Work out the finished part from the listing and answer in its coordinate system (mm). A direction names the side the tool comes from. Give positions to 0.01 mm unless a question says otherwise; leave off trailing zeros. Loops run counter-clockwise (first coordinate to the right, second up) from the corner with the lowest first, then second, coordinate; pieces in that order, holes last. Notation, with made-up numbers: M 26.5,33.5 L 61.5,33.5 A24 ccw 61.5,51.5 Z; hole C 34.5,2.25 d4. An arc over 180 degrees is marked long. Use a Markdown table: item, result.
Autodesk Inventor part; units mm, degrees
ref_plane "YZ Plane" through (0, 0, 0) normal (1, 0, 0) x (0, 1, 0)
ref_plane "XZ Plane" through (0, 0, 0) normal (0, 1, 0) x (-1, 0, 0)
ref_plane "XY Plane" through (0, 0, 0) normal (0, 0, 1) x (1, 0, 0)
sketch "Sketch1" plane through (0, 0, 0) normal (0, 0, 1) x (1, 0, 0)
  circle A0 centre (0, 0) radius 10.16
  line L0 (3.7395, -6.477) -> (-3.7395, -6.477)
  line L1 (-3.7395, -6.477) -> (-7.479, 0)
  line L2 (-7.479, 0) -> (-3.7395, 6.477)
  line L3 (-3.7395, 6.477) -> (3.7395, 6.477)
  line L4 (3.7395, 6.477) -> (7.479, 0)
  line L5 (7.479, 0) -> (3.7395, -6.477)
  dimension "d0" = 20.32
  dimension "d1" = 12.954
extrude "Extrusion1" add sketch "Sketch1" along normal blind 5.7112
properties part number "3DPRINT,KICKER,MOTOR,SPACER" material "ABS Plastic"
(1) The mould has two halves that part along X. Classify faces 3 (the flat face through (0, -7, 0)), 4 (the flat face through (-5.583, -3.284, 2.816)), 5 (the cylindrical face through (-1.323, -10.074, 2.816)), 6 (the flat face through (5.635, -3.193, 2.816)): released by +X, released by -X, zero draft, split by the parting line, or undercut.
Entries:
| item | result |
|---|---|
| face 3 | zero draft |
| face 4 | undercut |
| face 5 | split by the parting line |
| face 6 | undercut |
(2) Consider probe 1 along X at (y, z) = (1.75, 4.9); probe 2 along X at (y, z) = (-0.25, 0.5); probe 3 along Y at (x, z) = (6, 0.75). Determine where each line is inside the solid, lowest interval first. Write a range as [from, to].
Entries:
| item | result |
|---|---|
| probe 1 | x = [-10.01, -6.47], [6.47, 10.01] |
| probe 2 | x = [-10.16, -7.33], [7.33, 10.16] |
| probe 3 | y = [-8.2, -2.56], [2.56, 8.2] |
(3) Which of the six approach directions +Z, -Z, +X, -X, +Y, -Y give full straight-line access (tool end or side, diameter ignored) to faces 1 (the flat face through (-5.635, 3.193, 2.816)), 2 (the flat face through (0, -7, 5.711))?
Entries:
| item | result |
|---|---|
| face 1 | +Z, -Z |
| face 2 | +Z, +X, -X, +Y, -Y |
(4) Given P1, Ø2, axis at x = 3, z = 2, coming from the -Y side; P2, Ø4, axis at x = 3, y = -2.5, coming from the -Z side; P3, Ø1.5, axis at x = -4.5, z = 4, coming from the -Y side, each flat-ended and moving along its own axis, determine where each tip first touches the part or whether it passes through.
Entries:
| item | result |
|---|---|
| P1 | stops at y = -9.96 |
| P2 | passes through |
| P3 | stops at y = -9.44 |
(5) A cutting plane is placed at D-D (x = 9.25). Write down the section's boundary in (y, z), and give its area (3 significant figures).
Entries:
| item | result |
|---|---|
| outline | M -4.2,0 L 4.2,0 L 4.2,5.71 L -4.2,5.71 Z |
| area | 48.0 mm² |
(6) A cutting plane is placed at C-C (z = 2.8). Write down the section's boundary in (x, y).
Entries:
| item | result |
|---|---|
| outline | C 0,0 d20.32; hole M -7.48,0 L -3.74,-6.48 L 3.74,-6.48 L 7.48,0 L 3.74,6.48 L -3.74,6.48 Z |
(7) A cutting plane is placed at B-B (y = -4.5). Write down the section's boundary in (x, z).
Entries:
| item | result |
|---|---|
| outline | M -9.11,0 L -4.88,0 L -4.88,5.71 L -9.11,5.71 Z; M 4.88,0 L 9.11,0 L 9.11,5.71 L 4.88,5.71 Z |
(8) A cutting plane is placed at A-A (x = 0). Write down the section's boundary in (y, z).
Entries:
| item | result |
|---|---|
| outline | M -10.16,0 L -6.48,0 L -6.48,5.71 L -10.16,5.71 Z; M 6.48,0 L 10.16,0 L 10.16,5.71 L 6.48,5.71 Z |
